Work out the finished part from the listing and answer in its coordinate system (mm). A direction names the side the tool comes from. Coordinates: 2 decimals unless noted, no trailing zeros. Write item = value, one per line. Start each with the question number.
Q1. For a pull along X with two mould halves and no side action, classify faces 4 (the flat face through (2072.574, 1334, 1)), 5 (the flat face through (2104, 1326, 2)), 6 (the flat face through (2112.549, 1293.982, 0.986)), 7 (the flat face through (2130.977, 1325, 1)) as +X half, -X half, draft (parallel to the pull), parting line (faces both ways), or undercut.
Q2. Which of the six approach directions +Z, -Z, +X, -X, +Y, -Y give full straight-line access (tool end or side, diameter ignored) to faces 1 (the flat face through (2076, 1328.325, 1)), 2 (the flat face through (2119.69, 1344.53, 0.99)), 3 (the flat face through (2126.861, 1348.404, 0.986))?
Q3. The part is cut by section A-A, the plane z = 1.1. Count the separate pieces of the cut face and the enclosed holes in it, plus the area to 3 significant figures.
Q4. Straight lines are drawn through the part: L1, parallel to Y at x = 2121, z = 0.2; L2, parallel to X at y = 1311.5, z = 1.75; L3, parallel to X at y = 1346.5, z = 0.4. For each, find the intervals that lie inside material, in ascending order. Write a range as from..to.
Q5. A flat-ended cylindrical pin translates along its axis: pin 1 (0.6 mm diameter, centred on x = 2077, z = 1, fed in from -Y). Find the tip coordinate at first contact, or state that the pin passes through.
```python
from build123d import *

# Parameters (mm, degrees)
MODEL_R             = 1.5
MODEL_W             = 2
MODEL_H             = 10
BOSS_EXTRUDE2_DEPTH = 2


with BuildPart() as part:
    # Model → Boss-Extrude2 (new body)
    with BuildSketch(Plane.XY):
        with BuildLine():
            Line((2079.513177421, 1320.324687976), (2079.513177421, 1322.324687976))
            Line((2079.513177421, 1322.324687976), (2072.573837593, 1322.324687976))
            Line((2072.573837593, 1322.324687976), (2072.573837593, 1328.324687976))
            Line((2072.573837593, 1328.324687976), (2079.513177421, 1328.324687976))
            Line((2079.513177421, 1328.324687976), (2079.513177421, 1330.324687976))
            Line((2079.513177421, 1330.324687976), (2072.573837593, 1330.324687976))
            Line((2072.573837593, 1330.324687976), (2072.573837593, 1336.943408379))
            ThreePointArc((2072.573837593, 1336.943408379), (2074.982606168, 1342.074687976), (2078.222040366, 1346.726382553))
            Line((2078.222040366, 1346.726382553), (2083.954020375, 1350.035742754))
            Line((2083.954020375, 1350.035742754), (2087.423690289, 1344.026098178))
            Line((2087.423690289, 1344.026098178), (2089.155741097, 1345.026098178))
            Line((2089.155741097, 1345.026098178), (2085.686071183, 1351.035742754))
            Line((2085.686071183, 1351.035742754), (2090.882223605, 1354.035742754))
            Line((2090.882223605, 1354.035742754), (2094.351893519, 1348.026098178))
            Line((2094.351893519, 1348.026098178), (2096.083944327, 1349.026098178))
            Line((2096.083944327, 1349.026098178), (2092.614274413, 1355.035742754))
            Line((2092.614274413, 1355.035742754), (2098.346254422, 1358.345102956))
            ThreePointArc((2098.346254422, 1358.345102956), (2103.994457195, 1358.824687976), (2109.642659968, 1358.345102956))
            Line((2109.642659968, 1358.345102956), (2115.374639977, 1355.035742754))
            Line((2115.374639977, 1355.035742754), (2111.904970063, 1349.026098178))
            Line((2111.904970063, 1349.026098178), (2113.637020871, 1348.026098178))
            Line((2113.637020871, 1348.026098178), (2117.106690785, 1354.035742754))
            Line((2117.106690785, 1354.035742754), (2122.302843208, 1351.035742754))
            Line((2122.302843208, 1351.035742754), (2118.833173294, 1345.026098178))
            Line((2118.833173294, 1345.026098178), (2120.565224101, 1344.026098178))
            Line((2120.565224101, 1344.026098178), (2124.034894015, 1350.035742754))
            Line((2124.034894015, 1350.035742754), (2129.766874025, 1346.726382553))
            ThreePointArc((2129.766874025, 1346.726382553), (2133.006308222, 1342.074687976), (2135.415076798, 1336.943408379))
            Line((2135.415076798, 1336.943408379), (2135.415076798, 1313.705967573))
            ThreePointArc((2135.415076798, 1313.705967573), (2133.006308222, 1308.574687976), (2129.766874025, 1303.922993399))
            Line((2129.766874025, 1303.922993399), (2124.034894015, 1300.613633198))
            Line((2124.034894015, 1300.613633198), (2120.565224101, 1306.623277774))
            Line((2120.565224101, 1306.623277774), (2118.833173294, 1305.623277774))
            Line((2118.833173294, 1305.623277774), (2122.302843208, 1299.613633198))
            Line((2122.302843208, 1299.613633198), (2117.106690785, 1296.613633198))
            Line((2117.106690785, 1296.613633198), (2113.637020871, 1302.623277774))
            Line((2113.637020871, 1302.623277774), (2111.904970063, 1301.623277774))
            Line((2111.904970063, 1301.623277774), (2115.374639977, 1295.613633198))
            Line((2115.374639977, 1295.613633198), (2109.642659968, 1292.304272996))
            ThreePointArc((2109.642659968, 1292.304272996), (2103.994457195, 1291.824687976), (2098.346254422, 1292.304272996))
            Line((2098.346254422, 1292.304272996), (2092.614274413, 1295.613633198))
            Line((2092.614274413, 1295.613633198), (2096.083944327, 1301.623277774))
            Line((2096.083944327, 1301.623277774), (2094.351893519, 1302.623277774))
            Line((2094.351893519, 1302.623277774), (2090.882223605, 1296.613633198))
            Line((2090.882223605, 1296.613633198), (2085.686071183, 1299.613633198))
            Line((2085.686071183, 1299.613633198), (2089.155741097, 1305.623277774))
            Line((2089.155741097, 1305.623277774), (2087.423690289, 1306.623277774))
            Line((2087.423690289, 1306.623277774), (2083.954020375, 1300.613633198))
            Line((2083.954020375, 1300.613633198), (2078.222040366, 1303.922993399))
            ThreePointArc((2078.222040366, 1303.922993399), (2074.982606168, 1308.574687976), (2072.573837593, 1313.705967573))
            Line((2072.573837593, 1313.705967573), (2072.573837593, 1320.324687976))
            Line((2072.573837593, 1320.324687976), (2079.513177421, 1320.324687976))
        make_face()
        with Locations((2083.65962403, 1325.324687976)):
            Circle(MODEL_R, mode=Mode.SUBTRACT)
        with Locations((2093.827040613, 1342.935170078)):
            Circle(MODEL_R, mode=Mode.SUBTRACT)
        with Locations((2093.827040613, 1307.714205874)):
            Circle(MODEL_R, mode=Mode.SUBTRACT)
        with Locations((2114.161873777, 1307.714205874)):
            Circle(MODEL_R, mode=Mode.SUBTRACT)
        with Locations((2114.161873777, 1342.935170078)):
            Circle(MODEL_R, mode=Mode.SUBTRACT)
        with Locations((2078.013695082, 1340.324687976)):
            Circle(MODEL_R, mode=Mode.SUBTRACT)
        with Locations((2078.013695082, 1310.324687976)):
            Circle(MODEL_R, mode=Mode.SUBTRACT)
        with Locations((2129.975219309, 1340.324687976)):
            Circle(MODEL_R, mode=Mode.SUBTRACT)
        with Locations((2129.975219309, 1310.324687976)):
            Circle(MODEL_R, mode=Mode.SUBTRACT)
        with Locations((2129.976886457, 1325.324687976)):
            Rectangle(MODEL_W, MODEL_H, mode=Mode.SUBTRACT)
    extrude(amount=BOSS_EXTRUDE2_DEPTH)


solid = part.part
```
Model answer:
q1.face_4 = -X half
q1.face_5 = draft
q1.face_6 = +X half
q1.face_7 = undercut
q2.face_1 = +Z, -Z, -X
q2.face_2 = +Z, -Z
q2.face_3 = +Z, -Z, +X, +Y
q3.separate_pieces = 1
q3.enclosed_holes = 10
q3.area = 3,110 mm2
q4.L1 = 1298.86..1301.87, 1305.87..1344.78, 1348.78..1351.79
q4.L2 = 2073.48..2077.08, 2078.95..2129.04, 2130.91..2134.51
q4.L3 = 2078.04..2086, 2088.3..2119.68, 2121.99..2129.95
q5.pin_1 = 1305.08
